```python
from build123d import *

# Parameters (mm, degrees)
SKETCH_1_W              = 30
SKETCH_1_H              = 30
SKETCH_1_R              = 14
EXTRUDE_1_DEPTH         = 10
HOLE_WIZARD_3_5_3_5_1_D = 3.5


with BuildPart() as part:
    # Эскиз1 → Бобышка-Вытянуть1 (new body)
    with BuildSketch(Plane(origin=(0, 0, 0), x_dir=(1, 0, 0), z_dir=(0, 1, 0))):
        with Locations((15, 15)):
            Rectangle(SKETCH_1_W, SKETCH_1_H)
        with Locations(Location((15, 15, 0), (0, 0, 270))):
            Circle(SKETCH_1_R, mode=Mode.SUBTRACT)
    extrude(amount=EXTRUDE_1_DEPTH)

    # Диаметр отверстия Ø3.5 (3.5)1 (through all)
    with Locations(Plane(origin=(0, 10, 0), x_dir=(1, 0, 0), z_dir=(0, 1, 0))):
        with Locations((3, 27), (27, 27), (27, 3), (3, 3)):
            Hole(HOLE_WIZARD_3_5_3_5_1_D / 2)


solid = part.part
```
Input: part model. Units: mm. Frame: model coordinates. Give positions to 0.01 mm unless a question says otherwise; leave off trailing zeros. Order: outer loops, then holes, each group sorted by start corner. A loop starts at its lowest first (then second) coordinate and runs counter-clockwise, first axis right, second up.
1. Pin query (flat end, axial travel): pin 1 Ø2 at (x, z) = (23.5, -25) entering from -Y. Return the tip coordinate at first contact, or that it passes through.
Computed:
pin 1: stops at y = 0
2. Cut plane A-A (z = -10). Return loops of the section in (x, y), and give its area (3 significant figures).
Computed:
outline: (0, 0) - (1.92, 0) - (1.92, 10) - (0, 10) - close; (28.08, 0) - (30, 0) - (30, 10) - (28.08, 10) - close
area: 38.5 mm2
3. Cut plane C-C (y = 5.5). Return loops of the section in (x, z).
Computed:
outline: (0, -30) - (30, -30) - (30, 0) - (0, 0) - close; hole circle Ø28 at (15, -15); hole circle Ø3.5 at (3, -27); hole circle Ø3.5 at (3, -3); hole circle Ø3.5 at (27, -27); hole circle Ø3.5 at (27, -3)
4. Cut plane D-D (z = -27.5). Return loops of the section in (x, y), and give its area (3 significant figures).
Computed:
outline: (0, 0) - (1.32, 0) - (1.32, 10) - (0, 10) - close; (4.68, 0) - (8.7, 0) - (8.7, 10) - (4.68, 10) - close; (21.3, 0) - (25.32, 0) - (25.32, 10) - (21.3, 10) - close; (28.68, 0) - (30, 0) - (30, 10) - (28.68, 10) - close
area: 107 mm2
5. Draft query along X for faces 1 (the face through (30, 5, -15)), 2 (the face through (4, 0, -24)), 3 (the face through (28.75, 4.93, -27.08)). Return one class per face: released by +X, released by -X, zero draft, split by the parting line, or undercut.
Computed:
face 1: released by +X
face 2: zero draft
face 3: undercut
6. Cut plane B-B (x = 15). Return loops of the section in (y, z), and give its area (3 significant figures).
Computed:
outline: (0, -30) - (10, -30) - (10, -29) - (0, -29) - close; (0, -1) - (10, -1) - (10, 0) - (0, 0) - close
area: 20.0 mm2
7. Line query: probe 1 along Z at (x, y) = (3.25, 3); probe 2 along X at (y, z) = (5.5, -27); probe 3 along Z at (x, y) = (3, 7.5). Output: solid intervals per line, ascending.
Computed:
probe 1: z = -30 to -28.73, -25.27 to -22.61, -7.39 to -4.73, -1.27 to 0
probe 2: x = 0 to 1.25, 4.75 to 7.79, 22.21 to 25.25, 28.75 to 30
probe 3: z = -30 to -28.75, -25.25 to -22.21, -7.79 to -4.75, -1.25 to 0
